Autodesk Inventor part; units mm, degrees
ref_plane "YZ Plane" through (0, 0, 0) normal (1, 0, 0) x (0, 1, 0)
ref_plane "XZ Plane" through (0, 0, 0) normal (0, 1, 0) x (-1, 0, 0)
ref_plane "XY Plane" through (0, 0, 0) normal (0, 0, 1) x (1, 0, 0)
sketch "Sketch1" plane through (0, 0, 0) normal (0, 0, 1) x (1, 0, 0)
  circle A0 centre (0, 0) radius 1.5
  circle A1 centre (0, 0) radius 3.5
  circle A2 centre (0, 0) radius 5.75 construction
  line L0 (0, 0) -> (0, 5.75) construction
  circle A3 centre (0.5, 9.2365) radius 3.5
  line L1 (0, 0) -> (0, 5.75) construction
  line L2 (3.5, 0) -> (3.5, 5.75)
  line L3 (-3.5, 5.75) -> (-3.5, 0)
  arc A4 (-3.5, 0) -> (3.5, 0) centre (0, 0) ccw
  arc A5 (3.5, 5.75) -> (-1.9961, 2.875) centre (0, 5.75) ccw
  arc A6 (-3.4062, 0.805) -> (-3.4062, 4.945) centre (-12.1649, 2.875) ccw
  line L4 (0.5, 5.7365) -> (3.5, 5.7365)
  point P0 (0, 2.875)
  point P1 (-3.4345, 6.424)
  point P2 (3.5, 0)
  point P3 (3.244, 7.0639)
  point P4 (-3.5, 0)
  point P5 (-2.744, 7.9226)
  dimension "d2" = 11.5
  dimension "d3" = 7
  dimension "d0" = 3
  dimension "d1" = 7
  dimension "d4" = 3.5
  dimension "d9" = 0.5
  dimension "d10" = 9
extrude "Extrusion1" add sketch "Sketch1" along normal blind 4.7625 contours A1 | A1 A5 A3 L4 L2 | A1 A6 A5 | L3 A5 A6 A1
fillet "Fillet1" radius 1 1 edges at (-2.744, 7.9226, 2.3813)
fillet "Fillet2" radius 2 1 edges at (3.5, 5.7365, 2.3813)
sketch "Sketch2" plane through (0, 0, 0) normal (0, 0, -1) x (-1, 0, 0)
  line L0 (-3.5, 0) -> (-3.5, 3.7365)
  arc A0 (-3.5, 0) -> (3.5, 0) centre (0, 0) ccw
  circle A1 centre (0, 0) radius 1.5
  circle A2 centre (0, 0) radius 6.0263 construction
  arc A3 (3.4953, 5.9311) -> (1.8307, 6.6254) centre (2.4966, 5.8794) ccw
  arc A4 (-0.5, 5.7365) -> (1.8307, 6.6254) centre (-0.5, 9.2365) ccw
  line L1 (3.5, 5.75) -> (3.5, 0)
  line L2 (-1.5, 5.7365) -> (-0.5, 5.7365)
  arc A5 (-1.5, 5.7365) -> (-3.5, 3.7365) centre (-1.5, 3.7365) ccw
  arc A6 (-1.5, 5.7365) -> (-3.5, 3.7365) centre (-1.5, 3.7365) ccw
  arc A7 (3.5, 5.75) -> (3.4953, 5.9311) centre (0, 5.75) ccw
equation "\"d4\" = 0.5 * d1"
properties part number "Cam - Lever" material "Nylon 6/6"
Here's how the part is built. I have some questions about the finished solid (model axes, mm). A direction names the side the tool comes from. Round coordinates to 2 decimals unless told otherwise and drop trailing zeros. Order: outer loops, then holes, each group sorted by start corner. A loop starts at its lowest first (then second) coordinate and runs counter-clockwise, first axis right, second up. Notation, with made-up numbers: M 13,61.5 L 57,61.5 A21 ccw 57,91.5 Z; hole C 39,72 d3. An arc over 180 degrees is marked long. Answer in a Markdown table with one row per item.
Item 1: For faces 1 (the face through (1, 5.736, 2)), 2 (the face through (0.1, -3.5, 2.3)), which set-ups out of +Z, -Z, +X, -X, +Y, -Y let a thin tool reach every point of the face, with its end or its side?
A:
| item | result |
|---|---|
| face 1 | +Z, -Z, +X, +Y |
| face 2 | +Z, -Z, -Y |
Item 2: Imagine slicing it at D-D, the plane y = 4.75. Write out the boundary of the cut face in (x, z), and give its area (3 significant figures).
A:
| item | result |
|---|---|
| outline | M -3.5,0 L 3.22,0 L 3.22,4.76 L -3.5,4.76 Z |
| area | 32.0 mm2 |
Item 3: Imagine slicing it at C-C, the plane x = 2.25. Write out the boundary of the cut face in (y, z).
A:
| item | result |
|---|---|
| outline | M -2.68,0 L 5.59,0 L 5.59,4.76 L -2.68,4.76 Z |
Item 4: Thinking about a two-plate mould opening in Y: for faces 3 (the face through (-1.5, -0.07, 2.35)), 4 (the face through (-0.73, 5.96, 2.35)), 5 (the face through (-3.5, 3, 2)), which applies, +Y half, -Y half, draft (parallel to the pull), parting line (faces both ways), or undercut?
A:
| item | result |
|---|---|
| face 3 | undercut |
| face 4 | +Y half |
| face 5 | draft |
Item 5: If I drill on L1, parallel to X at y = -0.25, z = 2.9; L2, parallel to X at y = 1.25, z = 1.35; L3, parallel to Y at x = 0, z = 1.85, over which ranges is the centre line in solid material (lowest first)? Write a range as from..to.
A:
| item | result |
|---|---|
| L1 | x = -3.49..-1.48, 1.48..3.49 |
| L2 | x = -3.5..-0.83, 0.83..3.5 |
| L3 | y = -3.5..-1.5, 1.5..5.77 |
Item 6: I'm going to push flat-ended pins straight in: pin 1 (0.8 mm diameter, centred on x = 1, z = 2.5, fed in from +Y); pin 2 (1 mm diameter, centred on x = -2.5, y = -1, fed in from -Z); pin 3 (1 mm diameter, centred on x = -2, z = 1.5, fed in from -Y). Where does each tip first touch, or does it pass through?
A:
| item | result |
|---|---|
| pin 1 | stops at y = 5.74 |
| pin 2 | stops at z = 0 |
| pin 3 | stops at y = -3.16 |
Item 7: Imagine slicing it at A-A, the plane x = -1. Write out the boundary of the cut face in (y, z), and give its area (3 significant figures).
A:
| item | result |
|---|---|
| outline | M -3.35,0 L -1.12,0 L -1.12,4.76 L -3.35,4.76 Z; M 1.12,0 L 6.07,0 L 6.07,4.76 L 1.12,4.76 Z |
| area | 34.3 mm2 |
Item 8: Imagine slicing it at B-B, the plane y = -0.75. Write out the boundary of the cut face in (x, z), and give its area (3 significant figures).
A:
| item | result |
|---|---|
| outline | M -3.42,0 L -1.3,0 L -1.3,4.76 L -3.42,4.76 Z; M 1.3,0 L 3.42,0 L 3.42,4.76 L 1.3,4.76 Z |
| area | 20.2 mm2 |
